Read the model definition and answer for the solid it produces. Units are mm, in the model's axes. A direction names the side the tool comes from. Coordinates: 2 decimals unless noted, no trailing zeros. Write each loop counter-clockwise with the first axis right and the second up, starting at its lowest first coordinate (ties: lowest second). Pieces come first, ordered by that corner, then holes.
(1) The part is cut by section A-A, the plane x = 19.5. Determine the outline of the cut face in (y, z) (3 decimals).
(2) The part is cut by section B-B, the plane y = -17.5. Determine the outline of the cut face in (x, z), and give its area (3 significant figures).
(3) Given pin 1 (2 mm diameter, centred on x = 19.5, y = -33.77, fed in from -Z); pin 2 (3 mm diameter, centred on x = -9.5, z = 3.5, fed in from +Y); pin 3 (4 mm diameter, centred on x = 30, y = -51.96, fed in from +Z); pin 4 (1.5 mm diameter, centred on x = -45.96, y = 38.57, fed in from +Z), each flat-ended and moving along its own axis, determine where each tip first touches the part or whether it passes through.
(4) Which of the six approach directions +Z, -Z, +X, -X, +Y, -Y give full straight-line access (tool end or side, diameter ignored) to faces 1 (the cylindrical face through (-18.59, 35.21, 5.07)), 2 (the flat face through (22, -22, 17)), 3 (the flat face through (-20, 34, 12))?
(5) Straight lines are drawn through the part: line 1 along X through (y, z) = (33.5, 1.75); line 2 along X through (y, z) = (-20, 4.25); line 3 along Y through (x, z) = (-19.5, 6) (3 decimals). For each, find the intervals that lie inside material, in ascending order.
(6) The part is cut by section D-D, the plane x = 39. Determine the outline of the cut face in (y, z), and give its area (3 significant figures).
(7) The part is cut by section C-C, the plane z = 4.5. State how many separate pieces and enclosed holes the cut face has, and give its area (3 significant figures).
(8) Determine the mould class of faces 4 (the flat face through (30, -15, 0)), 5 (the cylindrical face through (47.69, 15.02, 14.46)), 6 (the flat face through (19, 34, 12)) for opening direction X: pulls with the +X half, pulls with the -X half, needs draft (parallel to the pull), parting line crosses it, or undercut.
```python
from build123d import *

# Parameters (mm, degrees)
SKETCH_R      = 70
SKETCH_R_2    = 30
SKETCH_R_3    = 1.25
PAD_DEPTH     = 12
SKETCH001_R   = 50
SKETCH001_R_2 = 30
SKETCH001_R_3 = 1.7
PAD001_DEPTH  = 5
SKETCH003_R   = 1.7
POCKET_DEPTH  = 10.001


with BuildPart() as part:
    # Sketch → Pad (new body)
    with BuildSketch(Plane.XY):
        Circle(SKETCH_R)
        Circle(SKETCH_R_2, mode=Mode.SUBTRACT)
        with Locations((-60, 0)):
            Circle(SKETCH_R_3, mode=Mode.SUBTRACT)
        with Locations((-45.962667, 38.567257)):
            Circle(SKETCH_R_3, mode=Mode.SUBTRACT)
        with Locations((-45.962667, -38.567257)):
            Circle(SKETCH_R_3, mode=Mode.SUBTRACT)
        with Locations((-10.418891, -59.088465)):
            Circle(SKETCH_R_3, mode=Mode.SUBTRACT)
        with Locations((30, -51.961524)):
            Circle(SKETCH_R_3, mode=Mode.SUBTRACT)
        with Locations((56.381557, -20.521209)):
            Circle(SKETCH_R_3, mode=Mode.SUBTRACT)
        with Locations((56.381557, 20.521209)):
            Circle(SKETCH_R_3, mode=Mode.SUBTRACT)
        with Locations((30, 51.961524)):
            Circle(SKETCH_R_3, mode=Mode.SUBTRACT)
        with Locations((-10.418891, 59.088465)):
            Circle(SKETCH_R_3, mode=Mode.SUBTRACT)
    extrude(amount=PAD_DEPTH)

    # Sketch001 (on Face13 of Pad) → Pad001 (join)
    with BuildSketch(Plane.XY.offset(12)):
        Circle(SKETCH001_R)
        Circle(SKETCH001_R_2, mode=Mode.SUBTRACT)
        with Locations((-19.5, 33.774991)):
            Circle(SKETCH001_R_3, mode=Mode.SUBTRACT)
        with Locations((19.5, 33.774991)):
            Circle(SKETCH001_R_3, mode=Mode.SUBTRACT)
        with Locations((39, 0)):
            Circle(SKETCH001_R_3, mode=Mode.SUBTRACT)
        with Locations((-39, 0)):
            Circle(SKETCH001_R_3, mode=Mode.SUBTRACT)
        with Locations((-19.5, -33.774991)):
            Circle(SKETCH001_R_3, mode=Mode.SUBTRACT)
        with Locations((19.5, -33.774991)):
            Circle(SKETCH001_R_3, mode=Mode.SUBTRACT)
    extrude(amount=PAD001_DEPTH)

    # Sketch003 → Pocket (cut, through all)
    with BuildSketch(Plane.XY.offset(10)):
        with Locations((-19.5, 33.774991)):
            Circle(SKETCH003_R)
        with Locations((19.5, 33.774991)):
            Circle(SKETCH003_R)
        with Locations((39, 0)):
            Circle(SKETCH003_R)
        with Locations((-39, 0)):
            Circle(SKETCH003_R)
        with Locations((-19.5, -33.774991)):
            Circle(SKETCH003_R)
        with Locations((19.5, -33.774991)):
            Circle(SKETCH003_R)
    extrude(amount=-POCKET_DEPTH, mode=Mode.SUBTRACT)


solid = part.part
```
Computed:
1. outline: (-67.229, 0) - (-35.475, 0) - (-35.475, 10) - (-32.075, 10) - (-32.075, 0) - (-22.798, 0) - (-22.798, 17) - (-32.075, 17) - (-32.075, 12) - (-35.475, 12) - (-35.475, 17) - (-46.041, 17) - (-46.041, 12) - (-67.229, 12) - close; (22.798, 0) - (32.075, 0) - (32.075, 10) - (35.475, 10) - (35.475, 0) - (67.229, 0) - (67.229, 12) - (46.041, 12) - (46.041, 17) - (35.475, 17) - (35.475, 12) - (32.075, 12) - (32.075, 17) - (22.798, 17) - close
2. outline: (-67.78, 0) - (-24.37, 0) - (-24.37, 17) - (-46.84, 17) - (-46.84, 12) - (-67.78, 12) - close; (24.37, 0) - (67.78, 0) - (67.78, 12) - (46.84, 12) - (46.84, 17) - (24.37, 17) - close
2. area: 1,270 mm2
3. pin 1: stops at z = 10
3. pin 2: stops at y = 69.54
3. pin 3: stops at z = 12
3. pin 4: passes through
4. face 1: -Z
4. face 2: +Z, +X, -X, +Y, -Y
4. face 3: +Z
5. line 1: x = -61.46 to -21.18, -17.82 to 17.82, 21.18 to 61.46
5. line 2: x = -67.08 to -22.36, 22.36 to 55.25, 57.52 to 67.08
5. line 3: y = -67.229 to -35.475, -32.075 to -22.798, 22.798 to 32.075, 35.475 to 67.229
6. outline: (-58.13, 0) - (-1.7, 0) - (-1.7, 10) - (1.7, 10) - (1.7, 0) - (58.13, 0) - (58.13, 12) - (31.29, 12) - (31.29, 17) - (1.7, 17) - (1.7, 12) - (-1.7, 12) - (-1.7, 17) - (-31.29, 17) - (-31.29, 12) - (-58.13, 12) - close
6. area: 1,660 mm2
7. separate pieces: 1
7. enclosed holes: 16
7. area: 12,500 mm2
8. face 4: needs draft
8. face 5: parting line crosses it
8. face 6: undercut
